Autodesk Inventor part; units mm, degrees
ref_plane "YZ Plane" through (0, 0, 0) normal (1, 0, 0) x (0, 1, 0)
ref_plane "XZ Plane" through (0, 0, 0) normal (0, 1, 0) x (-1, 0, 0)
ref_plane "XY Plane" through (0, 0, 0) normal (0, 0, 1) x (1, 0, 0)
sketch "Sketch1" plane through (0, 0, 0) normal (0, 0, 1) x (1, 0, 0)
  line L0 (-200, 100) -> (200, 100)
  line L1 (-200, -100) -> (-200, 100)
  line L2 (200, -100) -> (-200, -100)
  line L3 (121.9, 74) -> (121.9, 71)
  line L4 (171.9, 74) -> (121.9, 74)
  line L5 (171.9, 71) -> (171.9, 35.9)
  line L6 (121.9, 71) -> (171.9, 71)
  line L7 (121.9, 71) -> (121.9, 35.9)
  line L8 (171.9, 35.9) -> (121.9, 35.9)
  line L9 (171.9, 71) -> (171.9, 35.9)
  line L10 (171.9, 74) -> (171.9, 71)
  line L11 (121.9, 35.9) -> (171.9, 35.9)
  line L12 (171.9, 35.9) -> (171.9, 71)
  line L13 (171.9, 71) -> (121.9, 71)
  line L14 (121.9, 71) -> (121.9, 35.9)
  point P0 (0, 0)
extrude "Extrusion1" add sketch "Sketch1" along normal blind 3.175
sketch "Sketch2" plane through (0, 0, 3.175) normal (0, 0, 1) x (1, 0, 0)
  line L0 (171.9, 74) -> (121.9, 74)
  line L1 (171.9, 35.9) -> (171.9, 74)
  line L2 (121.9, 74) -> (171.9, 74)
  line L3 (171.9, 74) -> (171.9, 71)
  line L4 (121.9, 71) -> (121.9, 74)
  line L5 (121.9, 71) -> (121.9, 70.825)
  line L6 (121.9, 74) -> (121.9, 35.9)
  line L7 (121.9, 70.825) -> (171.9, 70.825)
  line L8 (171.9, 71) -> (171.9, 70.825)
  line L9 (171.9, 71) -> (171.9, 70.825)
  point P0 (0, 0)
  dimension "d3" = 3
  dimension "d54" = 0.175
extrude "Extrusion2" add sketch "Sketch2" along normal blind 34.925
sketch "Sketch3" plane through (121.9, 74, 0) normal (0, 1, 0) x (1, 0, 0)
  line L0 (50, 0) -> (0, 0)
  line L1 (0, 0) -> (0, -38.1)
  line L2 (50, -38.1) -> (0, -38.1)
  line L3 (50, 0) -> (50, -38.1)
  line L4 (50, -3.175) -> (50, -38.1)
  line L5 (0, -38.1) -> (0, -19.225)
  line L6 (50, -19.05) -> (60.9839, -19.05)
  line L7 (0, -38.1) -> (0, -22.1)
  line L8 (0, -22.1) -> (14, -22.1)
  line L9 (36, -22.1) -> (36, -22)
  point P0 (-121.9, 0)
  point P1 (14, -22)
  dimension "d55" = 16
sketch "Sketch4" plane through (121.9, 74, 0) normal (0, 1, 0) x (1, 0, 0)
  line L0 (50, 0) -> (0, 0)
  line L1 (0, 0) -> (0, -38.1)
  line L2 (50, -38.1) -> (0, -38.1)
  line L3 (50, 0) -> (50, -38.1)
  line L4 (0, -38.1) -> (0, -22.1)
  line L5 (25, -22) -> (25, -22)
  point P0 (-121.9, 0)
  dimension "d56" = 16
hole "Hole2" at (146.9, 74, 22) direction (0, -1, 0) diameter 8 end through all
hole "Hole3" at (135.9, 74, 22.1) at (157.9, 74, 22.1) direction (0, -1, 0) diameter 2 end through all
sketch "Sketch5" plane through (0, 0, 3.175) normal (0, 0, 1) x (1, 0, 0)
  line L0 (121.9, 70.825) -> (121.9, 35.9)
  line L1 (121.9, 35.9) -> (171.9, 35.9)
  line L2 (171.9, 35.9) -> (171.9, 70.825)
  line L3 (171.9, 70.825) -> (121.9, 70.825)
  line L4 (121.9, 35.9) -> (171.9, 35.9)
  line L5 (171.9, 35.9) -> (167.9, 35.9)
  line L6 (171.9, 35.9) -> (166.9, 35.9)
  circle A0 centre (166.9, 45.9) radius 1.5
  circle A1 centre (166.9, 60.9) radius 1.5
  circle A2 centre (126.9, 60.9) radius 1.5
  circle A3 centre (126.9, 45.9) radius 1.5
  line L7 (121.9, 35.9) -> (121.9, 45.9)
  point P0 (0, 0)
  dimension "d70" = 5
hole "Hole5" at (166.9, 45.9, 3.175) at (166.9, 60.9, 3.175) at (126.9, 60.9, 3.175) at (126.9, 45.9, 3.175) direction (0, 0, -1) diameter 3.18 end through all
properties part number "Suporte motor sensor"
Geometry: final body of the model. Coordinates: model frame, mm. A direction names the side the tool comes from. Give positions to 0.01 mm unless a question says otherwise; leave off trailing zeros. Loops run counter-clockwise (first coordinate to the right, second up) from the corner with the lowest first, then second, coordinate; pieces in that order, holes last. Notation, with made-up numbers: (40.25, 84.5) - (67.25, 84.5) arc R22 ccw to (67.25, 94.5) - close; hole circle Ø7 at (7.5, 50.5). An arc over 180 degrees is marked (long way). Answer as CSV lines item,"result". Start each with the question number.
1. Reachability of faces 4 (the face through (165.825, 62.072, 1.565)), 5 (the face through (147, 54, 3.175)) from +Z, -Z, +X, -X, +Y, -Y: full face, straight path, thin tool, end or side. Return the list, or none.
2. Ray query, L1, parallel to X at y = 60.9, z = 2.15; L2, parallel to Y at x = 126.9, z = 2.35; L3, parallel to X at y = 72, z = 22. Return the intervals inside material, ascending.
3. Draft query along X for faces 1 (the face through (147, 35.9, 2)), 2 (the face through (121.9, 63, 2)), 3 (the face through (158.876, 72.39, 21.883)). Return one class per face: released by +X, released by -X, zero draft, split by the parting line, or undercut.
4. Section B-B, the plane z = 22.1. Return loops of the section in (x, y) (3 decimals).
5. Pin query (flat end, axial travel): P1, Ø4, axis at x = 136.5, z = 5.5, coming from the -Y side (3 decimals); P2, Ø1.8, axis at x = 157.9, z = 22.1, coming from the +Y side; P3, Ø3.5, axis at x = 166.9, y = 45.9, coming from the +Z side (3 decimals). Return the tip coordinate at first contact, or that it passes through.
6. Section A-A, the plane x = 126.9. Return loops of the section in (y, z) (3 decimals).
7. Section C-C, the plane x = 146.9. Return loops of the section in (y, z) (3 decimals).
8. Section D-D, the plane y = 63.5. Return loops of the section in (x, z) (3 decimals), plus the area to 3 significant figures.
Answers:
1,face 4,"+Z, -Z"
1,face 5,"+Z, +X, -X, -Y"
2,L1,"x = 121.9 to 125.31, 128.49 to 165.31, 168.49 to 171.9"
2,L2,"y = 35.9 to 44.31, 47.49 to 59.31, 62.49 to 74"
2,L3,"x = 121.9 to 134.91, 136.89 to 142.9, 150.9 to 156.91, 158.89 to 171.9"
3,face 1,"zero draft"
3,face 2,"released by -X"
3,face 3,"undercut"
4,outline,"(121.9, 70.825) - (134.9, 70.825) - (134.9, 74) - (121.9, 74) - close; (136.9, 70.825) - (142.901, 70.825) - (142.901, 74) - (136.9, 74) - close; (150.899, 70.825) - (156.9, 70.825) - (156.9, 74) - (150.899, 74) - close; (158.9, 70.825) - (171.9, 70.825) - (171.9, 74) - (158.9, 74) - close"
5,P1,"stops at y = 70.825"
5,P2,"passes through"
5,P3,"stops at z = 3.175"
6,outline,"(35.9, 0) - (44.31, 0) - (44.31, 3.175) - (35.9, 3.175) - close; (47.49, 0) - (59.31, 0) - (59.31, 3.175) - (47.49, 3.175) - close; (62.49, 0) - (74, 0) - (74, 38.1) - (70.825, 38.1) - (70.825, 3.175) - (62.49, 3.175) - close"
7,outline,"(35.9, 0) - (74, 0) - (74, 18) - (70.825, 18) - (70.825, 3.175) - (35.9, 3.175) - close; (70.825, 26) - (74, 26) - (74, 38.1) - (70.825, 38.1) - close"
8,outline,"(121.9, 0) - (171.9, 0) - (171.9, 3.175) - (121.9, 3.175) - close"
8,area,"159 mm2"
